```python
from build123d import *

# Parameters (mm, degrees)
F0_R     = 2.45
F1_DEPTH = 6
F2_R     = 10
F3_DEPTH = 3
F4_W     = 3
F4_H     = 3
F5_DEPTH = 3.001


with BuildPart() as f1:
    # F0 (on Top) → F1 (new body)
    with BuildSketch(Plane.XY):
        with BuildLine():
            ThreePointArc((10.246951, -8), (12.292485, -4.230227), (13, 0))
            ThreePointArc((13, 0), (12.292485, 4.230227), (10.246951, 8))
            ThreePointArc((10.246951, 8), (0, 13), (-10.246951, 8))
            ThreePointArc((-10.246951, 8), (-13, 0), (-10.246951, -8))
            ThreePointArc((-10.246951, -8), (0, -13), (10.246951, -8))
        make_face()
        with BuildLine():
            ThreePointArc((10.246951, 8), (12.292485, 4.230227), (13, 0))
            ThreePointArc((13, 0), (12.292485, -4.230227), (10.246951, -8))
            Line((10.246951, -8), (32.370236, -8))
            Line((32.370236, -8), (32.370236, 8))
            Line((32.370236, 8), (10.246951, 8))
        make_face()
        with Locations((24.920236, 0)):
            Circle(F0_R, mode=Mode.SUBTRACT)
        with BuildLine():
            ThreePointArc((-10.246951, -8), (-13, 0), (-10.246951, 8))
            Line((-10.246951, 8), (-31.858318, 8))
            Line((-31.858318, 8), (-31.858318, -8))
            Line((-31.858318, -8), (-10.246951, -8))
        make_face()
        with Locations((-24.408318, 0)):
            Circle(F0_R, mode=Mode.SUBTRACT)
    extrude(amount=F1_DEPTH)

    # F2 (on face) → F3 (cut)
    with BuildSketch(Plane.XY.offset(6)):
        Circle(F2_R)
    extrude(amount=-F3_DEPTH, mode=Mode.SUBTRACT)

    # F4 (on face) → F5 (cut, through all)
    with BuildSketch(Plane.XY.offset(3)):
        with Locations((-7.998256, -0.119366)):
            Rectangle(F4_W, F4_H)
        Polygon((-4.593181, -4.874256), (-6.215104, -2.350495), (-8.738864, -3.972418), (-7.116942, -6.496178), align=None)
        Polygon((-1.230803, -6.582482), (-3.959699, -5.336237), (-5.205944, -8.065133), (-2.477048, -9.311378), align=None)
        Polygon((2.521346, -6.201695), (-0.448119, -6.62864), (-0.021174, -9.598104), (2.94829, -9.17116), align=None)
        Polygon((5.471985, -3.852792), (3.204737, -5.817374), (5.169319, -8.084623), (7.436567, -6.120041), align=None)
        Polygon((6.684308, -0.281532), (5.839111, -3.160011), (8.717589, -4.005209), (9.562787, -1.12673), align=None)
        Polygon((5.77341, 3.378234), (6.618608, 0.499755), (9.497087, 1.344952), (8.651889, 4.223431), align=None)
        Polygon((3.028496, 5.964556), (5.295744, 3.999974), (7.260327, 6.267223), (4.993078, 8.231805), align=None)
        Polygon((-0.678945, 6.656296), (2.290519, 6.229352), (2.717464, 9.198816), (-0.252001, 9.625761), align=None)
        Polygon((-4.171826, 5.233831), (-1.44293, 6.480076), (-2.689175, 9.208972), (-5.418071, 7.962727), align=None)
        Polygon((-6.341181, 2.148784), (-4.719259, 4.672544), (-7.243019, 6.294467), (-8.864942, 3.770706), align=None)
    extrude(amount=-F5_DEPTH, mode=Mode.SUBTRACT)


solid = f1.part
```
Source: CAD feature listing. Evaluate the final solid. Frame: model axes, mm. A direction names the side the tool comes from. Round coordinates to 2 decimals unless told otherwise and drop trailing zeros. Loops run counter-clockwise (first coordinate to the right, second up) from the corner with the lowest first, then second, coordinate; pieces in that order, holes last. Notation, with made-up numbers: (23, -30.75) - (60, -30.75) arc R13 ccw to (60, -18.75) - close; hole circle Ø1 at (55, 36). An arc over 180 degrees is marked (long way). Use CSV: the item, a comma, the result in double quotes.
Q1. Section query B-B, the plane z = 3.8. Output: boundary loops of the cut face in (x, y), then the cut area to 3 significant figures.
Reported:
outline,"(-31.86, -8) - (-10.25, -8) arc R13 ccw to (10.25, -8) - (32.37, -8) - (32.37, 8) - (10.25, 8) arc R13 ccw to (-10.25, 8) - (-31.86, 8) - close; hole circle Ø4.9 at (-24.41, 0); hole circle Ø20 at (0, 0); hole circle Ø4.9 at (24.92, 0)"
area,"819 mm^2"
Q2. Ray query, line 1 along Y through (x, z) = (1, 0.85); line 2 along Y through (x, z) = (-7, 2.55); line 3 along Y through (x, z) = (0, 3.95). Return the intervals inside material, ascending.
Reported:
line 1,"-12.96 to -9.45, -6.42 to 6.41, 9.45 to 12.96"
line 2,"-10.95 to -6.42, -2.85 to -1.62, 1.38 to 2.57, 6.14 to 10.95"
line 3,"-13 to -10, 10 to 13"
Q3. Section query C-C, the plane x = -19. Output: boundary loops of the cut face in (y, z), then the cut area to 3 significant figures.
Reported:
outline,"(-8, 0) - (8, 0) - (8, 6) - (-8, 6) - close"
area,"96.0 mm^2"
Q4. Section query A-A, the plane x = 4. Output: boundary loops of the cut face in (y, z).
Reported:
outline,"(-12.37, 0) - (-6.74, 0) - (-6.74, 3) - (-9.17, 3) - (-9.17, 6) - (-12.37, 6) - close; (-5.13, 0) - (5.12, 0) - (5.12, 3) - (-5.13, 3) - close; (7.09, 0) - (12.37, 0) - (12.37, 6) - (9.17, 6) - (9.17, 3) - (7.09, 3) - close"
Q5. Mould query, pull axis Y, two halves, no side actions, for faces 4 (the flat face through (7.233, 3.807, 1.521)), 5 (the flat face through (-31.858, 0, 3)), 6 (the flat face through (2.74, -7.71, 1.52)), 7 (the flat face through (-21, -8, 3)). Classes: pulls with the +Y half, pulls with the -Y half, needs draft (parallel to the pull), parting line crosses it, or undercut.
Reported:
face 4,"undercut"
face 5,"needs draft"
face 6,"undercut"
face 7,"pulls with the -Y half"
Q6. Pin query (flat end, axial travel): pin 1 Ø1 at (x, z) = (20, 3.5) entering from -Y; pin 2 Ø3 at (x, z) = (-23, 3) entering from +Y; pin 3 Ø3.5 at (x, z) = (-8.5, 1) entering from -Y; pin 4 Ø3 at (x, y) = (24.92, 0) entering from +Z. Return the tip coordinate at first contact, or that it passes through.
Reported:
pin 1,"y = -8"
pin 2,"y = 8"
pin 3,"y = -11.11"
pin 4,"through"
Q7. Reachability of faces 1 (the flat face through (21, 8, 3)), 2 (the flat face through (-2.576, -5.968, 1.521)), 3 (the flat face through (0, 0, 0)) from +Z, -Z, +X, -X, +Y, -Y: full face, straight path, thin tool, end or side. Return the list, or none.
Reported:
face 1,"+Z, -Z, +X, +Y"
face 2,"+Z, -Z"
face 3,"-Z, +X, -X, +Y, -Y"
